```python
from build123d import *

# Parameters (mm, degrees)
SKETCH1_R           = 1.65
BOSS_EXTRUDE1_DEPTH = 3
SKETCH3_W           = 3.5
SKETCH3_H           = 26
BOSS_EXTRUDE2_DEPTH = 14
SKETCH5_W           = 21.15
SKETCH5_H           = 8
SKETCH5_R           = 1.65
BOSS_EXTRUDE4_DEPTH = 3
SKETCH6_R           = 1.65
CUT_EXTRUDE1_DEPTH  = 42.674073475
FILLET1_R           = 10
FILLET2_R           = 2
SKETCH7_R           = 2.75
CUT_EXTRUDE2_DEPTH  = 4.1


with BuildPart() as part:
    # Sketch1 → Boss-Extrude1 (new body)
    with BuildSketch(Plane(origin=(0, 0, 0), x_dir=(1, 0, 0), z_dir=(0, 1, 0))):
        Polygon((0, 0), (25, 0), (25, -8), (20, -8), (20, -26), (0, -26), align=None)
        with Locations(Location((21.85, -3, 0), (0, 0, 270))):
            Circle(SKETCH1_R, mode=Mode.SUBTRACT)
    extrude(amount=BOSS_EXTRUDE1_DEPTH)

    # Sketch3 → Boss-Extrude2 (add)
    with BuildSketch(Plane(origin=(0, 3, 0), x_dir=(1, 0, 0), z_dir=(0, 1, 0))):
        with Locations((4.88, -13)):
            Rectangle(SKETCH3_W, SKETCH3_H)
    extrude(amount=BOSS_EXTRUDE2_DEPTH)

    # Sketch5 → Boss-Extrude4 (add)
    with BuildSketch(Plane(origin=(0, 3, 0), x_dir=(1, 0, 0), z_dir=(0, 1, 0))):
        with Locations((-10.575, -4)):
            Rectangle(SKETCH5_W, SKETCH5_H)
        with Locations(Location((-18.15, -3, 0), (0, 0, 270))):
            Circle(SKETCH5_R, mode=Mode.SUBTRACT)
    extrude(amount=-BOSS_EXTRUDE4_DEPTH)

    # Sketch6 → Cut-Extrude1 (cut, through all)
    with BuildSketch(Plane(origin=(6.63, 0, 0), x_dir=(0, 0, -1), z_dir=(1, 0, 0))):
        with Locations((-4, 11.25)):
            Circle(SKETCH6_R)
        with Locations((-22, 11.25)):
            Circle(SKETCH6_R)
    extrude(amount=-CUT_EXTRUDE1_DEPTH, mode=Mode.SUBTRACT)

    # Fillet1
    # the kernel refuses this fillet: 10 mm, written as the material it adds along each edge
    with BuildSketch(Plane(origin=(20, 0, 8), x_dir=(0, 0, 1), z_dir=(0, 1, 0))) as fillet1_piece_1:
        with BuildLine():
            CenterArc((8.660254038, 10), FILLET1_R, 210, 60)
            Line((0, 5), (-0.173205081, 4.9))
            ThreePointArc((-0.173205081, 4.9), (-0.2, 2.5), (-0.2, 0))
            Line((-0.2, 0), (0, -0.2))
            Line((0, -0.2), (8.660254038, -0.2))
            Line((8.660254038, -0.2), (8.660254038, 0))
        make_face()
    extrude(amount=3)
    with BuildSketch(Plane(origin=(0, 3, 8), x_dir=(0, 0, 1), z_dir=(0, -1, 0))) as fillet1_piece_2:
        with BuildLine():
            CenterArc((FILLET1_R, FILLET1_R), FILLET1_R, 180, 90)
            Line((0, FILLET1_R), (-FILLET1_R * 0.02, FILLET1_R))
            Line((-FILLET1_R * 0.02, FILLET1_R), (-FILLET1_R * 0.02, -FILLET1_R * 0.02))
            Line((-FILLET1_R * 0.02, -FILLET1_R * 0.02), (FILLET1_R, -FILLET1_R * 0.02))
            Line((FILLET1_R, -FILLET1_R * 0.02), (FILLET1_R, 0))
        make_face()
    extrude(amount=3)

    # Fillet2
    fillet2_edges = [part.edges().sort_by_distance(p)[0] for p in [
        (25, 1.5, 0),
        (25, 1.5, 8),
        (20, 1.5, 26),
        (0, 1.5, 26),
        (4.88, 17, 26),
        (4.88, 17, 0),
        (-21.15, 1.5, 8),
        (-21.15, 1.5, 0),
    ]]
    fillet(fillet2_edges, radius=FILLET2_R)

    # Sketch7 → Cut-Extrude2 (cut)
    with BuildSketch(Plane.XZ):
        with Locations(Location((3.153923281, 3, 0), (0, 0, 270))):
            Circle(SKETCH7_R)
    extrude(amount=-CUT_EXTRUDE2_DEPTH, mode=Mode.SUBTRACT)


solid = part.part
```
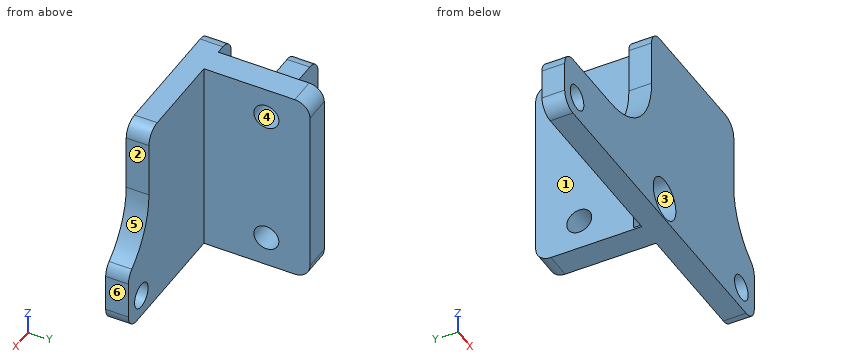
Check sheet for the modelled part. Datum: model origin and axes. Units: mm. Face numbers are marked on the shaded views. A direction names the side the tool comes from. Give positions to 0.01 mm unless a question says otherwise; leave off trailing zeros. Loops run counter-clockwise (first coordinate to the right, second up) from the corner with the lowest first, then second, coordinate; pieces in that order, holes last. Notation, with made-up numbers: M 58,-9 L 99,-9 A19 cw 99,17 Z; hole C -26,59.25 d6. An arc over 180 degrees is marked long. Answer as CSV lines item,"result".
Item 1: Scan lines: L1, parallel to X at y = 2.2, z = 3; L2, parallel to Y at x = 5.4, z = 22; L3, parallel to Y at x = 21, z = 7. Record each from-to range of solid material in increasing order.
Reply:
L1,"-21.15 to -19.8, -16.5 to 0.4, 5.9 to 20.2, 23.5 to 25"
L2,"0 to 9.6, 12.9 to 17"
L3,"0 to 3"
Item 2: Sectioned sample at C-C, the plane x = -18.15. Enter the section's corners in (y, z), then the cut area to 3 significant figures.
Reply:
outline,"M 0,0 L 3,0 L 3,1.35 L 0,1.35 Z; M 0,4.65 L 3,4.65 L 3,8 L 0,8 Z"
area,"14.1 mm^2"
Item 3: Sectioned sample at D-D, the plane z = 3.75. Enter the section's corners in (x, y), then the cut area to 3 significant figures.
Reply:
outline,"M -21.15,0 L -19.62,0 L -19.62,3 L -21.15,3 Z; M -16.68,0 L 0.51,0 L 0.51,3 L -16.68,3 Z; M 3.13,4.1 L 5.8,4.1 L 5.8,0 L 20.38,0 L 20.38,3 L 6.63,3 L 6.63,9.62 L 3.13,9.62 Z; M 3.13,12.88 L 6.63,12.88 L 6.63,17 L 3.13,17 Z; M 23.32,0 L 25,0 L 25,3 L 23.32,3 Z"
area,"140 mm^2"
Item 4: Depth check by flat-ended pin: pin 1 Ø1 at (x, z) = (19.5, 14.5) entering from +Y; pin 2 Ø8 at (y, z) = (13, 11) entering from -X; pin 3 Ø1.5 at (y, z) = (13.5, 10) entering from +X. Enter the tip coordinate at first touch or a pass-through.
Reply:
pin 1,"y = 3"
pin 2,"x = 3.13"
pin 3,"x = 6.63"
Item 5: Draft check along Z on the marked faces 4, 5 and 6. Enter one of: pulls with the +Z half, pulls with the -Z half, needs draft (parallel to the pull), parting line crosses it, or undercut.
Reply:
face 4,"undercut"
face 5,"pulls with the +Z half"
face 6,"needs draft"
Item 6: Set-up check for the marked faces 1, 2 and 3: record each of +Z, -Z, +X, -X, +Y, -Y from which the full face is reachable in a straight line by a thin tool's end or side.
Reply:
face 1,"+Z, -Z, -X, +Y"
face 2,"+Z, +X, +Y, -Y"
face 3,"-Y"
Item 7: Sectioned sample at B-B, the plane z = 22. Enter the section's corners in (x, y).
Reply:
outline,"M 0,0 L 20,0 L 20,3 L 6.63,3 L 6.63,9.6 L 3.13,9.6 L 3.13,3 L 0,3 Z; M 3.13,12.9 L 6.63,12.9 L 6.63,17 L 3.13,17 Z"
Item 8: Sectioned sample at A-A, the plane y = 11.25. Enter the section's corners in (x, z), then the cut area to 3 significant figures.
Reply:
outline,"M 3.13,0 L 6.63,0 L 6.63,2.35 L 3.13,2.35 Z; M 3.13,5.65 L 6.63,5.65 L 6.63,20.35 L 3.13,20.35 Z; M 3.13,23.65 L 6.63,23.65 L 6.63,26 L 3.13,26 Z"
area,"67.9 mm^2"
